from build123d import *

# Parameters (mm, degrees)
SKETCH_1_W          = 140
SKETCH_1_H          = 90
EXTRUDE_1_DEPTH     = 10
SKETCH_2_W          = 80
SKETCH_2_H          = 50
CUT_EXTRUDE_1_DEPTH = 4
SKETCH_3_W          = 90
SKETCH_3_H          = 6
EXTRUDE_2_DEPTH     = 15
SKETCH_4_W          = 6
SKETCH_4_H          = 80
EXTRUDE_3_DEPTH     = 15
SKETCH_5_R          = 10
EXTRUDE_4_DEPTH     = 20
SKETCH_6_R          = 15
EXTRUDE_5_DEPTH     = 25
SKETCH_7_R          = 4
CUT_EXTRUDE_2_DEPTH = 141
SKETCH_8_R          = 8
CUT_EXTRUDE_3_DEPTH = 20


with BuildPart() as part:
    # 草图1 → 凸台-拉伸1 (new body)
    with BuildSketch(Plane(origin=(0, 0, 0), x_dir=(1, 0, 0), z_dir=(0, 1, 0))):
        Rectangle(SKETCH_1_W, SKETCH_1_H)
    extrude(amount=EXTRUDE_1_DEPTH)

    # 草图2 → 切除-拉伸1 (cut)
    with BuildSketch(Plane(origin=(0, 0, 0), x_dir=(1, 0, 0), z_dir=(0, 1, 0))):
        Rectangle(SKETCH_2_W, SKETCH_2_H)
    extrude(amount=CUT_EXTRUDE_1_DEPTH, mode=Mode.SUBTRACT)

    # 草图3 → 凸台-拉伸2 (add)
    with BuildSketch(Plane(origin=(0, 10, 0), x_dir=(1, 0, 0), z_dir=(0, 1, 0))):
        Rectangle(SKETCH_3_W, SKETCH_3_H)
    extrude(amount=EXTRUDE_2_DEPTH)

    # 草图4 → 凸台-拉伸3 (add)
    with BuildSketch(Plane(origin=(0, 10, 0), x_dir=(1, 0, 0), z_dir=(0, 1, 0))):
        Rectangle(SKETCH_4_W, SKETCH_4_H)
    extrude(amount=EXTRUDE_3_DEPTH)

    # 草图5 → 凸台-拉伸4 (add)
    with BuildSketch(Plane(origin=(0, 10, 0), x_dir=(1, 0, 0), z_dir=(0, 1, 0))):
        with Locations(Location((-55, 32, 0), (0, 0, 90))):
            Circle(SKETCH_5_R)
        with Locations(Location((55, 32, 0), (0, 0, 90))):
            Circle(SKETCH_5_R)
        with Locations(Location((-55, -32, 0), (0, 0, 90))):
            Circle(SKETCH_5_R)
        with Locations(Location((55, -32, 0), (0, 0, 90))):
            Circle(SKETCH_5_R)
    extrude(amount=EXTRUDE_4_DEPTH)

    # 草图6 → 凸台-拉伸5 (add)
    with BuildSketch(Plane(origin=(0, 10, 0), x_dir=(1, 0, 0), z_dir=(0, 1, 0))):
        with Locations(Location((0, 0, 0), (0, 0, 78.463040967))):
            Circle(SKETCH_6_R)
    extrude(amount=EXTRUDE_5_DEPTH)

    # 草图7 → 切除-拉伸2 (cut, symmetric)
    with BuildSketch(Plane(origin=(0, 30, 0), x_dir=(1, 0, 0), z_dir=(0, 1, 0))):
        with Locations(Location((-55, 32, 0), (0, 0, 270))):
            Circle(SKETCH_7_R)
        with Locations(Location((55, 32, 0), (0, 0, 270))):
            Circle(SKETCH_7_R)
        with Locations(Location((-55, -32, 0), (0, 0, 270))):
            Circle(SKETCH_7_R)
        with Locations(Location((55, -32, 0), (0, 0, 270))):
            Circle(SKETCH_7_R)
    extrude(amount=CUT_EXTRUDE_2_DEPTH, both=True, mode=Mode.SUBTRACT)

    # 草图8 → 切除-拉伸3 (cut)
    with BuildSketch(Plane(origin=(0, 35, 0), x_dir=(1, 0, 0), z_dir=(0, 1, 0))):
        with Locations(Location((0, 0, 0), (0, 0, 270))):
            Circle(SKETCH_8_R)
    extrude(amount=-CUT_EXTRUDE_3_DEPTH, mode=Mode.SUBTRACT)


solid = part.part
Input: part model. Units: mm. Frame: model coordinates. A direction names the side the tool comes from. Coordinates: 2 decimals unless noted, no trailing zeros. Write each loop counter-clockwise with the first axis right and the second up, starting at its lowest first coordinate (ties: lowest second). Pieces come first, ordered by that corner, then holes. Notation, with made-up numbers: M -38,-26.75 L 4,-26.75 A9 ccw 4,-14.75 Z; hole C -7.75,87 d8. An arc over 180 degrees is marked long. Answer as a JSON object with one key per item and string values. Group by question number.
(1) Section A-A on y = 20. Give the number of separate pieces and of enclosed holes in the cut face, plus the area to 3 significant figures.
(2) Ray query, line 1 along X through (y, z) = (15.5, -32); line 2 along X through (y, z) = (6.5, 32); line 3 along X through (y, z) = (20, 35.5). Return the intervals inside material, ascending. Write a range as [from, to].
(3) Section C-C on z = -32. Output: boundary loops of the cut face in (x, y), plus the area to 3 significant figures.
(4) Mould query, pull axis X, two halves, no side actions, for faces 1 (the face through (-40, 2, 0)), 2 (the face through (13.7, 22.32, 6.11)), 3 (the face through (-45, 17, 0)). Classes: pulls with the +X half, pulls with the -X half, needs draft (parallel to the pull), parting line crosses it, or undercut.
(5) Section D-D on y = 6.5. Output: boundary loops of the cut face in (x, z), plus the area to 3 significant figures.
(6) Set-up query: faces 4 (the face through (-30, 17, -3)), 5 (the face through (3, 17, -27)), 6 (the face through (-30, 17, 3)), 7 (the face through (-45.24, 19.86, 34.17)), 8 (the face through (40, 2, 0)). Return all of +Z, -Z, +X, -X, +Y, -Y with unobstructed straight access to the full face (end or side cutting, diameter ignored); none if empty.
(7) Section B-B on x = -55. Output: boundary loops of the cut face in (y, z).
(8) Contact query for flat-ended pins moving along their axis: P1, Ø12, axis at y = 21, z = -22.5, coming from the +X side; P2, Ø16, axis at x = 50.5, z = 36, coming from the +Y side; P3, Ø10, axis at y = 26, z = 7.5, coming from the +X side. Output: stop coordinate, or through.
Result set:
{
 "1": {"separate pieces": "5", "enclosed holes": "5", "area": "2,220 mm2"},
 "2": {"line 1": "x = [-65, -59], [-51, -45], [-3, 3], [45, 51], [59, 65]", "line 2": "x = [-70, -59], [-51, 51], [59, 70]", "line 3": "x = [-64.37, -56.94], [-53.06, -45.63], [-3, 3], [45.63, 53.06], [56.94, 64.37]"},
 "3": {"outline": "M -70,0 L -59,0 L -59,30 L -65,30 L -65,10 L -70,10 Z; M -51,0 L 51,0 L 51,30 L 45,30 L 45,10 L 3,10 L 3,25 L -3,25 L -3,10 L -45,10 L -45,30 L -51,30 Z; M 59,0 L 70,0 L 70,10 L 65,10 L 65,30 L 59,30 Z", "area": "1,810 mm2"},
 "4": {"face 1": "undercut", "face 2": "parting line crosses it", "face 3": "pulls with the -X half"},
 "5": {"outline": "M -70,-45 L 70,-45 L 70,45 L -70,45 Z; hole C -55,-32 d8; hole C -55,32 d8; hole C 55,-32 d8; hole C 55,32 d8", "area": "12,400 mm2"},
 "6": {"face 4": "-Z, -X, +Y", "face 5": "-Z, +Y", "face 6": "+Z, -X, +Y", "face 7": "+Y", "face 8": "-Y"},
 "7": {"outline": "M 0,-45 L 10,-45 L 10,-42 L 30,-42 L 30,-36 L 0,-36 Z; M 0,-28 L 30,-28 L 30,-22 L 10,-22 L 10,22 L 30,22 L 30,28 L 0,28 Z; M 0,36 L 30,36 L 30,42 L 10,42 L 10,45 L 0,45 Z"},
 "8": {"P1": "stops at x = 64.37", "P2": "stops at y = 30", "P3": "stops at x = 45"}
}
